```python
from build123d import *

# Parameters (mm, degrees)
SKETCH1_W           = 38.1
SKETCH1_H           = 38.1
SKETCH1_R           = 1.143
BOSS_EXTRUDE1_DEPTH = 1.6764
BOSS_EXTRUDE2_DEPTH = 3.429
SKETCH3_R           = 7.366
BOSS_EXTRUDE3_DEPTH = 6.985
SKETCH4_R           = 5.969
BOSS_EXTRUDE4_DEPTH = 1.905
SKETCH5_R           = 6.985
BOSS_EXTRUDE5_DEPTH = 3.6322
SKETCH6_R           = 4.064
CUT_EXTRUDE1_DEPTH  = 0.254
SKETCH7_W           = 10.033
SKETCH7_H           = 4.7244
SKETCH7_W_2         = 8.763
SKETCH7_H_2         = 3.4544
BOSS_EXTRUDE6_DEPTH = 6.604
CUT_EXTRUDE2_REACH  = 41.725
SKETCH9_W           = 3.175
SKETCH9_H           = 6.604


with BuildPart() as part:
    # Sketch1 → Boss-Extrude1 (new body)
    with BuildSketch(Plane(origin=(0, 0, 0), x_dir=(1, 0, 0), z_dir=(0, 1, 0))):
        Rectangle(SKETCH1_W, SKETCH1_H)
        with Locations(Location((-13.97, 13.97, 0), (0, 0, 270))):
            Circle(SKETCH1_R, mode=Mode.SUBTRACT)
        with Locations(Location((-13.97, -13.97, 0), (0, 0, 270))):
            Circle(SKETCH1_R, mode=Mode.SUBTRACT)
        with Locations(Location((13.97, -13.97, 0), (0, 0, 270))):
            Circle(SKETCH1_R, mode=Mode.SUBTRACT)
        with Locations(Location((13.97, 13.97, 0), (0, 0, 270))):
            Circle(SKETCH1_R, mode=Mode.SUBTRACT)
    extrude(amount=BOSS_EXTRUDE1_DEPTH)

    # Sketch2 → Boss-Extrude2 (add)
    with BuildSketch(Plane(origin=(0, 1.6764, 0), x_dir=(1, 0, 0), z_dir=(0, 1, 0))):
        with BuildLine():
            Line((-8.5725, -1.905), (-8.5725, -8.5725))
            Line((-8.5725, -8.5725), (8.5725, -8.5725))
            Line((8.5725, -8.5725), (8.5725, -1.905))
            ThreePointArc((8.5725, -1.905), (10.4775, 0), (8.5725, 1.905))
            Line((8.5725, 1.905), (8.5725, 8.5725))
            Line((8.5725, 8.5725), (-8.5725, 8.5725))
            Line((-8.5725, 8.5725), (-8.5725, 1.905))
            ThreePointArc((-8.5725, 1.905), (-10.4775, 0), (-8.5725, -1.905))
        make_face()
    extrude(amount=BOSS_EXTRUDE2_DEPTH)

    # Sketch3 → Boss-Extrude3 (add)
    with BuildSketch(Plane(origin=(0, 5.1054, 0), x_dir=(1, 0, 0), z_dir=(0, 1, 0))):
        with Locations(Location((0, 0, 0), (0, 0, 270))):
            Circle(SKETCH3_R)
    extrude(amount=BOSS_EXTRUDE3_DEPTH)

    # Sketch4 → Boss-Extrude4 (add)
    with BuildSketch(Plane(origin=(0, 12.0904, 0), x_dir=(1, 0, 0), z_dir=(0, 1, 0))):
        with Locations(Location((0, 0, 0), (0, 0, 90))):
            Circle(SKETCH4_R)
    extrude(amount=BOSS_EXTRUDE4_DEPTH)

    # Sketch5 → Boss-Extrude5 (add)
    with BuildSketch(Plane(origin=(0, 13.9954, 0), x_dir=(1, 0, 0), z_dir=(0, 1, 0))):
        with Locations(Location((0, 0, 0), (0, 0, 270))):
            Circle(SKETCH5_R)
    extrude(amount=BOSS_EXTRUDE5_DEPTH)

    # Sketch6 → Cut-Extrude1 (cut)
    with BuildSketch(Plane(origin=(0, 17.6276, 0), x_dir=(1, 0, 0), z_dir=(0, 1, 0))):
        with Locations(Location((0, 0, 0), (0, 0, 270))):
            Circle(SKETCH6_R)
    extrude(amount=-CUT_EXTRUDE1_DEPTH, mode=Mode.SUBTRACT)

    # Sketch7 → Boss-Extrude6 (add)
    with BuildSketch(Plane.XZ):
        with Locations((-6.2865, -13.3858)):
            Rectangle(SKETCH7_W, SKETCH7_H)
        with Locations((-6.2865, -13.3858)):
            Rectangle(SKETCH7_W_2, SKETCH7_H_2, mode=Mode.SUBTRACT)
    extrude(amount=BOSS_EXTRUDE6_DEPTH)

    # Sketch9 → Cut-Extrude2 (cut, up to next)
    with BuildSketch(Plane.XY.offset(-11.0236), mode=Mode.PRIVATE) as cut_extrude2_sk1:
        with Locations((-6.2865, -3.302)):
            Rectangle(SKETCH9_W, SKETCH9_H)
    cut_extrude2_tool1 = extrude(cut_extrude2_sk1.sketch, amount=-CUT_EXTRUDE2_REACH, mode=Mode.PRIVATE) & part.part
    add(cut_extrude2_tool1.solids().sort_by_distance((-6.2865, -3.302, -11.0236))[0], mode=Mode.SUBTRACT)


solid = part.part
```
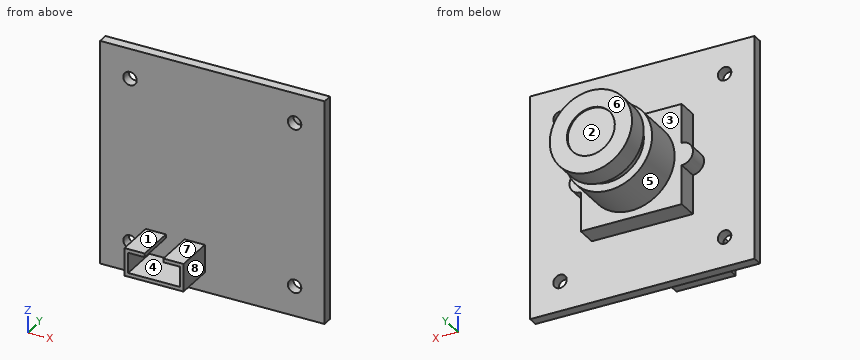
Verification items for the finished model (mm, model axes). Face numbers are marked on the shaded views. A direction names the side the tool comes from. Round coordinates to 2 decimals unless told otherwise and drop trailing zeros. Order: outer loops, then holes, each group sorted by start corner. A loop starts at its lowest first (then second) coordinate and runs counter-clockwise, first axis right, second up.
1) Depth check by flat-ended pin: pin 1 (8 mm diameter, centred on x = 9.5, y = 6, fed in from -Z); pin 2 (12 mm diameter, centred on x = 12.5, y = 10.5, fed in from -Z); pin 3 (8 mm diameter, centred on x = -1.5, y = 12.5, fed in from +Z); pin 4 (1 mm diameter, centred on y = -2, z = 4, fed in from -X). Enter the tip coordinate at first touch or a pass-through.
Geometry says:
pin 1: stops at z = -8.57
pin 2: stops at z = -3.47
pin 3: stops at z = 7.37
pin 4: passes through
2) Cross-section at A-A, the plane x = -13.97. Record the cut outline in (y, z), plus the area to 3 significant figures.
Geometry says:
outline: (0, -19.05) - (1.68, -19.05) - (1.68, -15.11) - (0, -15.11) - close; (0, -12.83) - (1.68, -12.83) - (1.68, 12.83) - (0, 12.83) - close; (0, 15.11) - (1.68, 15.11) - (1.68, 19.05) - (0, 19.05) - close
area: 56.2 mm2
3) Cross-section at B-B, the plane z = 13.97. Record the cut outline in (x, y), plus the area to 3 significant figures.
Geometry says:
outline: (-19.05, 0) - (-15.11, 0) - (-15.11, 1.68) - (-19.05, 1.68) - close; (-12.83, 0) - (12.83, 0) - (12.83, 1.68) - (-12.83, 1.68) - close; (15.11, 0) - (19.05, 0) - (19.05, 1.68) - (15.11, 1.68) - close
area: 56.2 mm2
4) Draft check along Z on the marked faces 1, 2, 3 and 4. Enter one of: +Z half, -Z half, draft (parallel to the pull), parting line (faces both ways), or undercut.
Geometry says:
face 1: +Z half
face 2: undercut
face 3: draft
face 4: undercut
5) Cross-section at D-D, the plane y = -4.5. Record the cut outline in (x, z) (3 decimals), plus the area to 3 significant figures.
Geometry says:
outline: (-11.303, -15.748) - (-1.27, -15.748) - (-1.27, -11.024) - (-4.699, -11.024) - (-4.699, -11.659) - (-1.905, -11.659) - (-1.905, -15.113) - (-10.668, -15.113) - (-10.668, -11.659) - (-7.874, -11.659) - (-7.874, -11.024) - (-11.303, -11.024) - close
area: 15.1 mm2
6) Material ranges on line 1 (X direction, y = 1, z = -13.97); line 2 (Y direction, x = -3, z = -10); line 3 (Z direction, x = -2.5, y = 2.5), recorded low to high.
Geometry says:
line 1: x = -19.05 to -15.11, -12.83 to 12.83, 15.11 to 19.05
line 2: y = 0 to 1.68
line 3: z = -8.57 to 8.57
7) Tool access check on the marked faces 5, 6, 7 and 8. Record the directions out of +Z, -Z, +X, -X, +Y, -Y that give a thin tool (end or side, any length) a straight path to the whole face; none if there is none.
Geometry says:
face 5: +Y
face 6: +Z, -Z, +X, -X, +Y
face 7: +Z, +X, -X, -Y
face 8: +Z, -Z, +X, -Y
